For this review, use the dimensioned drawing (mm, ordinates from the lowest corner) and the shaded views. A direction names the side the tool comes from. Give positions to 0.01 mm unless a question says otherwise; leave off trailing zeros. Loops run counter-clockwise (first coordinate to the right, second up) from the corner with the lowest first, then second, coordinate; pieces in that order, holes last. Notation, with made-up numbers: M 65.25,-29 L 82.25,-29 A13 ccw 82.25,-12 Z; hole C 24.25,33.25 d1. An arc over 180 degrees is marked long. Use CSV: the item, a comma, the result in double quotes. Start each with the question number.
1. The part is to be moulded in two halves that separate along Y. For the marked faces 3, 4, 5 and 6, say which applies: pulls with the +Y half, pulls with the -Y half, needs draft (parallel to the pull), parting line crosses it, or undercut.
2. Take a section at B-B, the plane x = 23. Write out the cut boundary in (y, z), and give its area (3 significant figures).
3. To check wall thickness, follow line 1 (Z direction, x = 7, y = 34.9); line 2 (X direction, y = 35.45, z = 5); line 3 (X direction, y = 35.9, z = 21) (3 decimals). State the ranges of each line that lie inside material, in increasing order. Write a range as [from, to].
4. Take a section at C-C, the plane y = 14. Write out the cut boundary in (x, z), and give its area (3 significant figures).
5. Tool access review of the marked faces 1 and 2: name each direction out of +Z, -Z, +X, -X, +Y, -Y from which nothing blocks a thin tool from reaching the whole face with its end or side.
6. Take a section at D-D, the plane z = 21. Write out the cut boundary in (x, y), and give its area (3 significant figures).
7. Take a section at A-A, the plane x = 15. Write out the cut boundary in (y, z), and give its area (3 significant figures).
8. Insertion check: P1, Ø2.5, axis at x = 23, z = 21, coming from the +Y side; P2, Ø4, axis at x = 12, z = 21, coming from the -Y side; P3, Ø5, axis at y = 13, z = 4.5, coming from the -X side. Each pin has a flat end and moves straight along its axis. Give the tip position at first contact, or say it passes through.
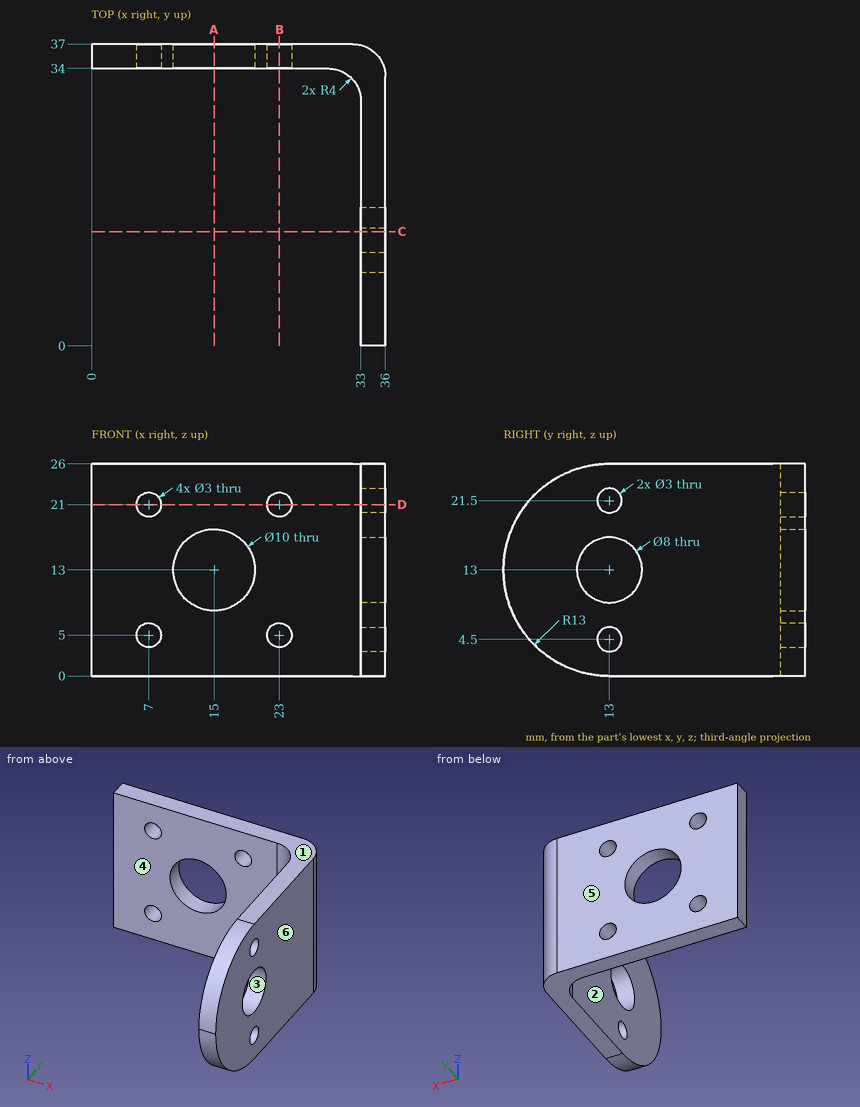
Result set:
1,face 3,"undercut"
1,face 4,"pulls with the -Y half"
1,face 5,"pulls with the +Y half"
1,face 6,"needs draft"
2,outline,"M 34,0 L 37,0 L 37,3.5 L 34,3.5 Z; M 34,6.5 L 37,6.5 L 37,19.5 L 34,19.5 Z; M 34,22.5 L 37,22.5 L 37,26 L 34,26 Z"
2,area,"60.0 mm2"
3,line 1,"[0, 3.5], [6.5, 19.5], [22.5, 26]"
3,line 2,"[0, 5.5], [8.5, 21.5], [24.5, 35.16]"
3,line 3,"[0, 5.5], [8.5, 21.5], [24.5, 34.755]"
4,outline,"M 33,0 L 36,0 L 36,3.38 L 33,3.38 Z; M 33,5.62 L 36,5.62 L 36,9.13 L 33,9.13 Z; M 33,16.87 L 36,16.87 L 36,20.38 L 33,20.38 Z; M 33,22.62 L 36,22.62 L 36,26 L 33,26 Z"
4,area,"41.3 mm2"
5,face 1,"+Z, +X, -X, +Y, -Y"
5,face 2,"+Z, -Z, -X, -Y"
6,outline,"M 0,34 L 5.5,34 L 5.5,37 L 0,37 Z; M 8.5,34 L 21.5,34 L 21.5,37 L 8.5,37 Z; M 24.5,34 L 29,34 A4 cw 33,30 L 33,14.41 L 36,14.41 L 36,33 A4 ccw 32,37 L 24.5,37 Z; M 33,2.75 L 36,2.75 L 36,11.59 L 33,11.59 Z"
6,area,"175 mm2"
7,outline,"M 34,0 L 37,0 L 37,8 L 34,8 Z; M 34,18 L 37,18 L 37,26 L 34,26 Z"
7,area,"48.0 mm2"
8,P1,"through"
8,P2,"y = 34"
8,P3,"x = 33"
